from build123d import *

# Parameters (mm, degrees)
EXTRUDE_3_DEPTH     = 550
SKETCH_2_R          = 2.2
SKETCH_2_W          = 8.2
SKETCH_2_H          = 14
CUT_EXTRUDE_1_DEPTH = 8.148528137


with BuildPart() as part:
    # Эскиз1 → Вытянуть-Тонкостенный3 (new body)
    with BuildSketch(Plane(origin=(0, 0, 0), x_dir=(0, 0, -1), z_dir=(1, 0, 0))):
        with BuildLine():
            Line((6.3, 11.5), (5.501920783, 10.701920783))
            Line((5.501920783, 10.701920783), (4.371381229, 10.701920783))
            Line((4.371381229, 10.701920783), (3.573302011, 11.5))
            Line((3.573302011, 11.5), (1, 11.5))
            ThreePointArc((1, 11.5), (0.292893219, 11.207106781), (0, 10.5))
            Line((0, 10.5), (0, -10.5))
            ThreePointArc((0, -10.5), (0.292893219, -11.207106781), (1, -11.5))
            Line((1, -11.5), (3.573302011, -11.5))
            Line((3.573302011, -11.5), (4.371381229, -10.701920783))
            Line((4.371381229, -10.701920783), (5.501920783, -10.701920783))
            Line((5.501920783, -10.701920783), (6.3, -11.5))
            Line((6.3, -11.5), (7.148528137, -10.651471863))
            Line((7.148528137, -10.651471863), (5.998977057, -9.501920783))
            Line((5.998977057, -9.501920783), (3.874324954, -9.501920783))
            Line((3.874324954, -9.501920783), (3.076245737, -10.3))
            Line((3.076245737, -10.3), (1.2, -10.3))
            Line((1.2, -10.3), (1.2, 10.3))
            Line((1.2, 10.3), (3.076245737, 10.3))
            Line((3.076245737, 10.3), (3.874324954, 9.501920783))
            Line((3.874324954, 9.501920783), (5.998977057, 9.501920783))
            Line((5.998977057, 9.501920783), (7.148528137, 10.651471863))
            Line((7.148528137, 10.651471863), (6.3, 11.5))
        make_face()
    extrude(amount=EXTRUDE_3_DEPTH)

    # Эскиз2 → Вырез-Вытянуть1 (cut, through all)
    with BuildSketch(Plane.XY):
        with Locations((499.6, 0)):
            Circle(SKETCH_2_R)
        with Locations((276.6, 0)):
            Circle(SKETCH_2_R)
        with Locations((83.6, 0)):
            Circle(SKETCH_2_R)
        with Locations((545.9, 0)):
            Rectangle(SKETCH_2_W, SKETCH_2_H)
        with BuildLine():
            Line((522, 2.2), (527, 2.2))
            ThreePointArc((527, 2.2), (529.2, 0), (527, -2.2))
            Line((527, -2.2), (522, -2.2))
            ThreePointArc((522, -2.2), (519.8, 0), (522, 2.2))
        make_face()
        with BuildLine():
            Line((506.4, 1.779598361), (506.4, -2.5))
            ThreePointArc((506.4, -2.5), (508.6, -4.7), (510.8, -2.5))
            Line((510.8, -2.5), (510.8, 1.779598361))
            ThreePointArc((510.8, 1.779598361), (508.6, 3.979598361), (506.4, 1.779598361))
        make_face()
        with BuildLine():
            Line((283.4, 1.779598361), (283.4, -2.5))
            ThreePointArc((283.4, -2.5), (285.6, -4.7), (287.8, -2.5))
            Line((287.8, -2.5), (287.8, 1.779598361))
            ThreePointArc((287.8, 1.779598361), (285.6, 3.979598361), (283.4, 1.779598361))
        make_face()
        with BuildLine():
            Line((299, -2.2), (304, -2.2))
            ThreePointArc((304, -2.2), (306.2, 0), (304, 2.2))
            Line((304, 2.2), (299, 2.2))
            ThreePointArc((299, 2.2), (296.8, 0), (299, -2.2))
        make_face()
        with BuildLine():
            Line((94.8, -2.5), (94.8, 1.779598361))
            ThreePointArc((94.8, 1.779598361), (92.6, 3.979598361), (90.4, 1.779598361))
            Line((90.4, 1.779598361), (90.4, -2.5))
            ThreePointArc((90.4, -2.5), (92.6, -4.7), (94.8, -2.5))
        make_face()
        with BuildLine():
            Line((106, 2.2), (111, 2.2))
            ThreePointArc((111, 2.2), (113.2, 0), (111, -2.2))
            Line((111, -2.2), (106, -2.2))
            ThreePointArc((106, -2.2), (103.8, 0), (106, 2.2))
        make_face()
    extrude(amount=-CUT_EXTRUDE_1_DEPTH, mode=Mode.SUBTRACT)


solid = part.part
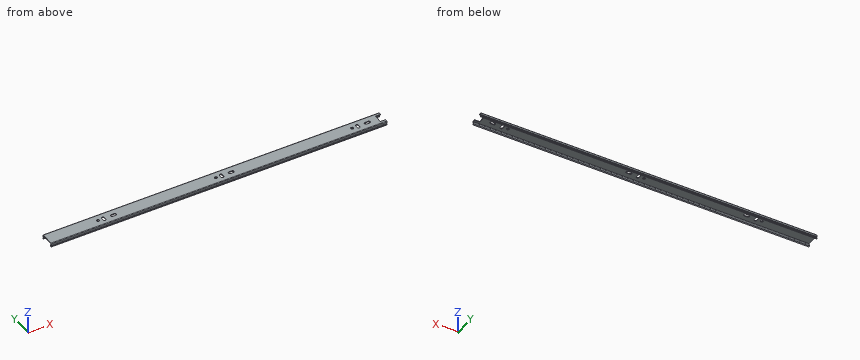
Verification items for the finished model (mm, model axes). Give positions to 0.01 mm unless a question says otherwise; leave off trailing zeros. Write each loop counter-clockwise with the first axis right and the second up, starting at its lowest first coordinate (ties: lowest second). Pieces come first, ordered by that corner, then holes. Notation, with made-up numbers: M -40,42 L -12,42 A27 cw -12,58 Z; hole C 75.5,85.25 d11. An arc over 180 degrees is marked long. Put each result on its own line as item: value. Start each with the question number.
1. Scan lines: line 1 along Y through (x, z) = (316, -2); line 2 along X through (y, z) = (3, -1); line 3 along Y through (x, z) = (83.6, -0.7). Record each from-to range of solid material in increasing order. Write a range as [from, to].
2. Go/stop test with flat-tipped pins: pin 1 Ø0.6 at (x, z) = (274.5, -5) entering from -Y; pin 2 Ø3.5 at (x, y) = (499.6, 0) entering from +Z; pin 3 Ø0.6 at (x, z) = (280, -5) entering from +Y; pin 4 Ø2 at (y, z) = (1, -1) entering from +X. Record where each tip stops, or that it passes through.
3. Section check A-A (x = 164). Record the cut outline in (y, z).
Answer list:
1. line 1: [-11.5, -10.3], [10.3, 11.5]
1. line 2: [0, 90.77], [94.43, 283.77], [287.43, 506.77], [510.43, 541.8]
1. line 3: [-11.45, -2.2], [2.2, 11.45]
2. pin 1: y = -10.7
2. pin 2: through
2. pin 3: y = 10.7
2. pin 4: x = 541.8
3. outline: M -11.5,-6.3 L -10.65,-7.15 L -9.5,-6 L -9.5,-3.87 L -10.3,-3.08 L -10.3,-1.2 L 10.3,-1.2 L 10.3,-3.08 L 9.5,-3.87 L 9.5,-6 L 10.65,-7.15 L 11.5,-6.3 L 10.7,-5.5 L 10.7,-4.37 L 11.5,-3.57 L 11.5,-1 A1 ccw 10.5,0 L -10.5,0 A1 ccw -11.5,-1 L -11.5,-3.57 L -10.7,-4.37 L -10.7,-5.5 Z
